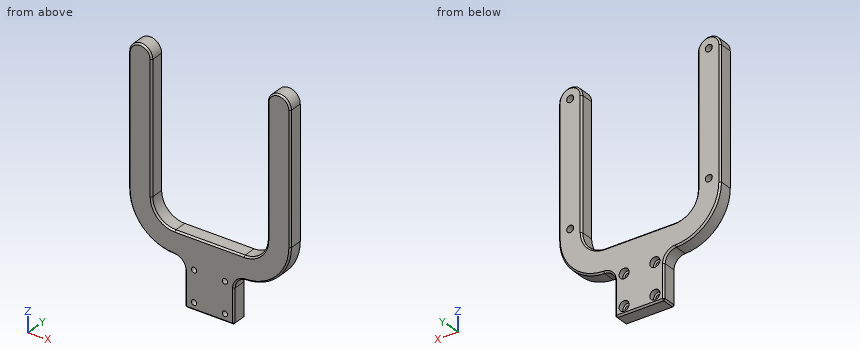
from build123d import *

# Parameters (mm, degrees)
SKETCH1_R                                           = 2.25
BOSS_EXTRUDE1_DEPTH                                 = 10
FILLET1_R                                           = 7.5
CHAMFER1_SIZE                                       = 1
SKETCH5_R                                           = 2.25
BOSS_EXTRUDE2_DEPTH                                 = 4
CBORE_FOR_M3_HEX_SOCKET_HEAD_CAP_SCREW1_D           = 3.4
CBORE_FOR_M3_HEX_SOCKET_HEAD_CAP_SCREW1_CBORE_D     = 6.5
CBORE_FOR_M3_HEX_SOCKET_HEAD_CAP_SCREW1_CBORE_DEPTH = 3.4


with BuildPart() as part:
    # Sketch1 → Boss-Extrude1 (new body)
    with BuildSketch(Plane(origin=(0, 0, 0), x_dir=(1, 0, 0), z_dir=(0, 1, 0))):
        with BuildLine():
            Line((0, 57.25), (22.5, 57.25))
            ThreePointArc((22.5, 57.25), (33.106601718, 52.856601718), (37.5, 42.25))
            Line((37.5, 42.25), (37.5, -42.25))
            ThreePointArc((37.5, -42.25), (45, -49.75), (52.5, -42.25))
            Line((52.5, -42.25), (52.5, 42.25))
            ThreePointArc((52.5, 42.25), (43.713203436, 63.463203436), (22.5, 72.25))
            Line((22.5, 72.25), (16, 72.25))
            Line((16, 72.25), (16, 102.25))
            Line((16, 102.25), (0, 102.25))
            Line((0, 102.25), (0, 57.25))
        make_face()
        with Locations((45, -42.25)):
            Circle(SKETCH1_R, mode=Mode.SUBTRACT)
        with Locations((45, 37.75)):
            Circle(SKETCH1_R, mode=Mode.SUBTRACT)
    extrude(amount=BOSS_EXTRUDE1_DEPTH)

    # Fillet1
    fillet1_edges = [part.edges().sort_by_distance(p)[0] for p in [
        (16, 5, -72.25),
    ]]
    fillet(fillet1_edges, radius=FILLET1_R)

    # Chamfer1
    chamfer1_edges = [part.edges().sort_by_distance(p)[0] for p in [
        (8, 0, -102.25),
        (43.99418526, 0, -63.178449536),
        (52.5, 0, 0),
        (45, 0, 49.75),
        (37.5, 0, 0),
        (33.106601718, 10, -52.856601718),
        (33.106601718, 0, -52.856601718),
        (11.25, 0, -57.25),
        (37.5, 10, 0),
        (16, 5, -102.25),
        (45, 10, 49.75),
        (52.5, 10, 0),
        (43.99418526, 10, -63.178449536),
        (16, 0, -90.993332148),
        (16, 10, -90.993332148),
        (8, 10, -102.25),
        (18.126453685, 0, -74.504551911),
        (18.126453685, 10, -74.504551911),
        (11.25, 10, -57.25),
    ]]
    chamfer(chamfer1_edges, length=CHAMFER1_SIZE)

    # Sketch5 → Boss-Extrude2 (add)
    with BuildSketch(Plane.XZ):
        with Locations((45, -37.75)):
            Circle(SKETCH5_R)
        with Locations((45, 42.25)):
            Circle(SKETCH5_R)
    extrude(amount=-BOSS_EXTRUDE2_DEPTH)

    # Mirror1: part across plane


with BuildPart() as part_1:
    add(part.part)
    add(part.part.mirror(Plane(origin=(0, 10, -57.25), x_dir=(0, 0, 1), z_dir=(1, 0, 0))))

    # CBORE for M3 Hex Socket Head Cap Screw1 (through all)
    with Locations(Plane(origin=(0, 10, 0), x_dir=(1, 0, 0), z_dir=(0, 1, 0))):
        with Locations((10, 97.25), (-10, 97.25), (-10, 77.25), (10, 77.25)):
            CounterBoreHole(CBORE_FOR_M3_HEX_SOCKET_HEAD_CAP_SCREW1_D / 2, CBORE_FOR_M3_HEX_SOCKET_HEAD_CAP_SCREW1_CBORE_D / 2, CBORE_FOR_M3_HEX_SOCKET_HEAD_CAP_SCREW1_CBORE_DEPTH)


solid = part_1.part
Work out the finished part from the listing and answer in its coordinate system (mm). Give positions to 0.01 mm unless a question says otherwise; leave off trailing zeros. Loops run counter-clockwise (first coordinate to the right, second up) from the corner with the lowest first, then second, coordinate; pieces in that order, holes last. Notation, with made-up numbers: (54, 34) - (112, 34) arc R14 cw to (112, 61) - close; hole circle Ø9 at (-15, 64). An arc over 180 degrees is marked (long way). Answer in a Markdown table with one row per item.
(1) Section D-D (z = -77.25) is taken. State how many separate pieces and enclosed holes the cut face has, and give its area (3 significant figures).
Results list:
| item | result |
|---|---|
| separate pieces | 3 |
| enclosed holes | 0 |
| area | 237 mm² |
(2) Consider L1, parallel to X at y = 6.1, z = 42.25; L2, parallel to Z at x = 10, y = 8.05; L3, parallel to Z at x = -10, y = 4.75. Determine where each line is inside the solid, lowest interval first. Write a range as [from, to].
Results list:
| item | result |
|---|---|
| L1 | x = [-52.5, -47.25], [-42.75, -37.5], [37.5, 42.75], [47.25, 52.5] |
| L2 | z = [-102.25, -100.5], [-94, -80.5], [-74, -57.25] |
| L3 | z = [-102.25, -98.95], [-95.55, -78.95], [-75.55, -57.25] |
(3) Section B-B (z = -97.25) is taken. Give the vertices of the cut face in (x, y).
Results list:
| item | result |
|---|---|
| outline | (-16, 1) - (-15, 0) - (-11.7, 0) - (-11.7, 6.6) - (-13.25, 6.6) - (-13.25, 10) - (-15, 10) - (-16, 9) - close; (-8.3, 0) - (8.3, 0) - (8.3, 6.6) - (6.75, 6.6) - (6.75, 10) - (-6.75, 10) - (-6.75, 6.6) - (-8.3, 6.6) - close; (11.7, 0) - (15, 0) - (16, 1) - (16, 9) - (15, 10) - (13.25, 10) - (13.25, 6.6) - (11.7, 6.6) - close |
(4) Flat-ended cylindrical pins translate along their axes: pin 1 Ø5 at (x, y) = (40.5, 8.5) entering from -Z; pin 2 Ø2 at (x, z) = (-44.5, -38) entering from +Y; pin 3 Ø6 at (x, y) = (7, 6) entering from +Z. Find the tip coordinate at first contact, or state that the pin passes through.
Results list:
| item | result |
|---|---|
| pin 1 | stops at z = -67.94 |
| pin 2 | stops at y = 4 |
| pin 3 | stops at z = -57.25 |
(5) Section A-A (z = -37.75) is taken. Give the vertices of the cut face in (x, y), and give its area (3 significant figures).
Results list:
| item | result |
|---|---|
| outline | (-52.5, 1) - (-51.5, 0) - (-38.5, 0) - (-37.5, 1) - (-37.5, 9) - (-38.5, 10) - (-42.75, 10) - (-42.75, 4) - (-47.25, 4) - (-47.25, 10) - (-51.5, 10) - (-52.5, 9) - close; (37.5, 1) - (38.5, 0) - (51.5, 0) - (52.5, 1) - (52.5, 9) - (51.5, 10) - (47.25, 10) - (47.25, 4) - (42.75, 4) - (42.75, 10) - (38.5, 10) - (37.5, 9) - close |
| area | 242 mm² |
(6) Section C-C (z = 37) is taken. Give the vertices of the cut face in (x, y).
Results list:
| item | result |
|---|---|
| outline | (-52.5, 1) - (-51.5, 0) - (-38.5, 0) - (-37.5, 1) - (-37.5, 9) - (-38.5, 10) - (-51.5, 10) - (-52.5, 9) - close; (37.5, 1) - (38.5, 0) - (51.5, 0) - (52.5, 1) - (52.5, 9) - (51.5, 10) - (38.5, 10) - (37.5, 9) - close |
